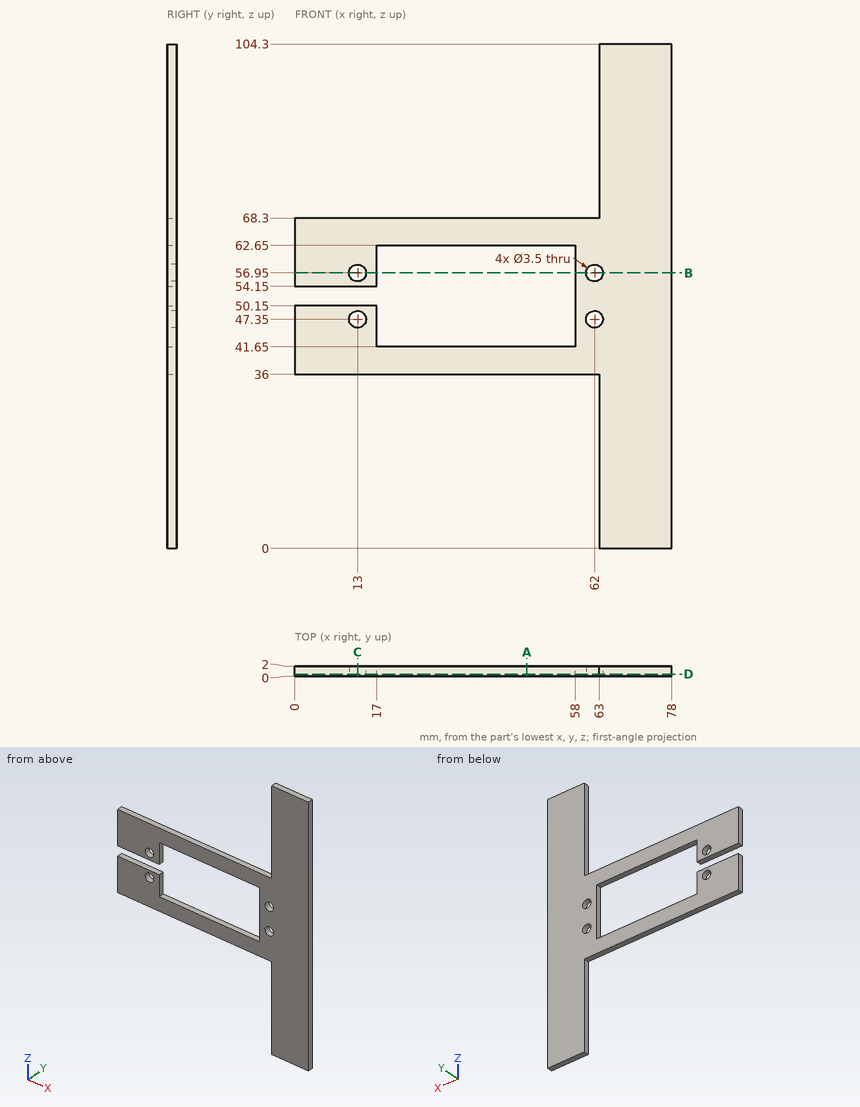
Study the drawing (mm; zero at the part's minimum x, y, z) and answer. Coordinates: 2 decimals unless noted, no trailing zeros. Order: outer loops, then holes, each group sorted by start corner. A loop starts at its lowest first (then second) coordinate and runs counter-clockwise, first axis right, second up. Notation, with made-up numbers: (-16, 27.5) -> (18, 27.5) arc R29 ccw to (18, 60.5) -> close; hole circle Ø6 at (-28, 35). An arc over 180 degrees is marked (long way). Answer in a Markdown table with one row per item. Add a question column.
Item 1: Find section D-D (y = 0.4). Write down the section's boundary in (x, z), then the cut area to 3 significant figures.
Item 2: Find the intervals of material crossed by L1, parallel to Z at x = 62, y = 1.25; L2, parallel to X at y = 0.65, z = 56.95; L3, parallel to Z at x = 13, y = 1.3, in increasing order. Write a range as from..to.
Item 3: Find section B-B (z = 56.95). Write down the section's boundary in (x, y), then the cut area to 3 significant figures.
Item 4: Find section A-A (x = 48). Write down the section's boundary in (y, z).
Item 5: Each of these flat-tipped pins is pushed along its axis until it touches: P1, Ø0.6, axis at y = 1.5, z = 89.5, coming from the -X side; P2, Ø1, axis at x = 30.5, y = 1, coming from the -Z side; P3, Ø0.6, axis at x = 45.5, y = 1.5, coming from the +Z side. Where does it stop, or does it pass through?
Item 6: Find section C-C (x = 13). Write down the section's boundary in (y, z), then the cut area to 3 significant figures.
Result set:
| question | item | result |
|---|---|---|
| 1 | outline | (0, 36) -> (63, 36) -> (63, 0) -> (78, 0) -> (78, 104.3) -> (63, 104.3) -> (63, 68.3) -> (0, 68.3) -> (0, 54.15) -> (17, 54.15) -> (17, 62.65) -> (58, 62.65) -> (58, 41.65) -> (17, 41.65) -> (17, 50.15) -> (0, 50.15) -> close; hole circle Ø3.5 at (13, 47.35); hole circle Ø3.5 at (13, 56.95); hole circle Ø3.5 at (62, 47.35); hole circle Ø3.5 at (62, 56.95) |
| 1 | area | 2,630 mm² |
| 2 | L1 | z = 36..45.6, 49.1..55.2, 58.7..68.3 |
| 2 | L2 | x = 0..11.25, 14.75..17, 58..60.25, 63.75..78 |
| 2 | L3 | z = 36..45.6, 49.1..50.15, 54.15..55.2, 58.7..68.3 |
| 3 | outline | (0, 0) -> (11.25, 0) -> (11.25, 2) -> (0, 2) -> close; (14.75, 0) -> (17, 0) -> (17, 2) -> (14.75, 2) -> close; (58, 0) -> (60.25, 0) -> (60.25, 2) -> (58, 2) -> close; (63.75, 0) -> (78, 0) -> (78, 2) -> (63.75, 2) -> close |
| 3 | area | 60.0 mm² |
| 4 | outline | (0, 36) -> (2, 36) -> (2, 41.65) -> (0, 41.65) -> close; (0, 62.65) -> (2, 62.65) -> (2, 68.3) -> (0, 68.3) -> close |
| 5 | P1 | stops at x = 63 |
| 5 | P2 | stops at z = 36 |
| 5 | P3 | stops at z = 68.3 |
| 6 | outline | (0, 36) -> (2, 36) -> (2, 45.6) -> (0, 45.6) -> close; (0, 49.1) -> (2, 49.1) -> (2, 50.15) -> (0, 50.15) -> close; (0, 54.15) -> (2, 54.15) -> (2, 55.2) -> (0, 55.2) -> close; (0, 58.7) -> (2, 58.7) -> (2, 68.3) -> (0, 68.3) -> close |
| 6 | area | 42.6 mm² |
